Geometry check sheet. Reference: drawing and pictorial views, mm from the part's lowest x, y, z. A direction names the side the tool comes from. Round coordinates to 2 decimals unless told otherwise and drop trailing zeros. Write each loop counter-clockwise with the first axis right and the second up, starting at its lowest first coordinate (ties: lowest second). Pieces come first, ordered by that corner, then holes.
Item 1: Material ranges on line 1 along Y through (x, z) = (63, 4.75); line 2 along X through (y, z) = (5.75, 6.25); line 3 along X through (y, z) = (5.5, 2.75), recorded low to high.
Item 2: Section check B-B, the plane y = 17.25. Record the cut outline in (x, z).
Item 3: Set-up check for the marked faces 1, 2 and 3: record each of +Z, -Z, +X, -X, +Y, -Y from which the full face is reachable in a straight line by a thin tool's end or side.
Item 4: Depth check by flat-ended pin: pin 1 (4.5 mm diameter, centred on y = 15, z = 4, fed in from +X); pin 2 (2.5 mm diameter, centred on x = 49.5, z = 5.5, fed in from +Y). Enter the tip coordinate at first touch or a pass-through.
Item 5: Section check D-D, the plane x = 15.5. Record the cut outline in (y, z).
Item 6: Section check A-A, the plane x = 75. Record the cut outline in (y, z).
Item 7: Release check for a two-part mould opening along X. For the marked faces 4, 5 and 6 record: pulls with the +X half, pulls with the -X half, needs draft (parallel to the pull), parting line crosses it, or undercut.
Item 8: Section check C-C, the plane y = 6. Record the cut outline in (x, z).
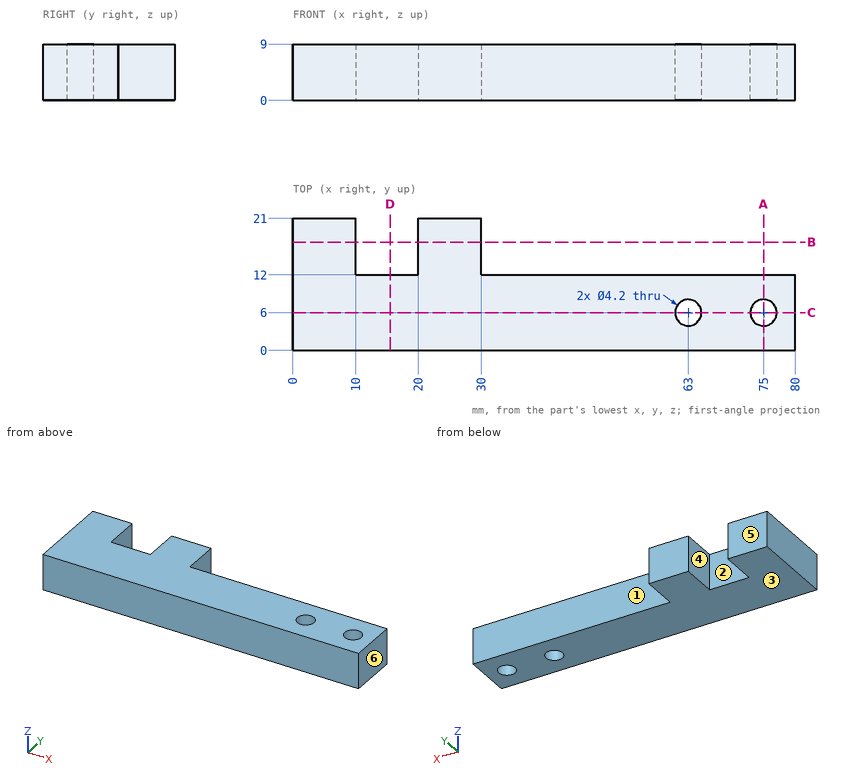
Values found:
1. line 1: y = 0 to 3.9, 8.1 to 12
1. line 2: x = 0 to 60.91, 65.09 to 72.91, 77.09 to 80
1. line 3: x = 0 to 60.96, 65.04 to 72.96, 77.04 to 80
2. outline: (0, 0) - (10, 0) - (10, 9) - (0, 9) - close; (20, 0) - (30, 0) - (30, 9) - (20, 9) - close
3. face 1: +Z, -Z, +X, +Y
3. face 2: +Z, -Z, +Y
3. face 3: -Z, +X, -X, +Y, -Y
4. pin 1: stops at x = 30
4. pin 2: stops at y = 12
5. outline: (0, 0) - (12, 0) - (12, 9) - (0, 9) - close
6. outline: (0, 0) - (3.9, 0) - (3.9, 9) - (0, 9) - close; (8.1, 0) - (12, 0) - (12, 9) - (8.1, 9) - close
7. face 4: undercut
7. face 5: needs draft
7. face 6: pulls with the +X half
8. outline: (0, 0) - (60.9, 0) - (60.9, 9) - (0, 9) - close; (65.1, 0) - (72.9, 0) - (72.9, 9) - (65.1, 9) - close; (77.1, 0) - (80, 0) - (80, 9) - (77.1, 9) - close
